The model under review builds one solid part; all positions refer to its coordinate system, in mm. Round coordinates to 2 decimals unless told otherwise and drop trailing zeros. Write each loop counter-clockwise with the first axis right and the second up, starting at its lowest first coordinate (ties: lowest second). Pieces come first, ordered by that corner, then holes. Notation, with made-up numbers: (-36.5, 46.25) -> (-15.5, 46.25) arc R16 ccw to (-15.5, 75.25) -> close; hole circle Ø1 at (-21.75, 8). An arc over 180 degrees is marked (long way). Use CSV: the item, a comma, the result in double quotes. Start each with the question number.
1) Take a section at B-B, the plane x = 504. Give the boundary of the cut face in (y, z).
2) For pin 1 Ø4 at (x, y) = (20, 60) entering from -Z; pin 2 Ø7 at (x, y) = (517, 269) entering from +Z; pin 3 Ø5 at (x, y) = (91, 15) entering from +Z; pin 4 Ø5.5 at (x, y) = (375, 15) entering from +Z, all flat-tipped, find the tip position at first contact; note any pin that passes through.
3) Wall thickness on probe 1 along X at (y, z) = (231.5, 0.6); probe 2 along Y at (x, z) = (20, 0.35); probe 3 along X at (y, z) = (224, 0.6): over which ranges is each line inside the solid? List them lowest first. Write a range as [from, to].
4) Take a section at A-A, the plane y = 205.5. Give the boundary of the cut face in (x, z), then the cut area to 3 significant figures.
from build123d import *

# Parameters (mm, degrees)
SKETCH_1_W                  = 750
SKETCH_1_H                  = 284
SKETCH_1_W_2                = 320
SKETCH_1_H_2                = 220
SKETCH_1_W_3                = 20
EXTRUDE_1_DEPTH             = 3
HOLE_WIZARD_M41_AT_2_COUNT  = 2
HOLE_WIZARD_M41_AT_2_PITCH  = 254
HOLE_WIZARD_M41_AT_3_COUNT  = 2
HOLE_WIZARD_M41_AT_3_PITCH  = 71
HOLE_WIZARD_M41_AT_4_COUNT  = 2
HOLE_WIZARD_M41_AT_4_PITCH  = 263.736611035
HOLE_WIZARD_M41_AT_5_COUNT  = 2
HOLE_WIZARD_M41_AT_5_PITCH  = 142
HOLE_WIZARD_M41_AT_6_COUNT  = 2
HOLE_WIZARD_M41_AT_6_PITCH  = 290.998281782
HOLE_WIZARD_M41_AT_7_COUNT  = 2
HOLE_WIZARD_M41_AT_7_PITCH  = 213
HOLE_WIZARD_M41_AT_8_COUNT  = 2
HOLE_WIZARD_M41_AT_8_PITCH  = 331.489064676
HOLE_WIZARD_M41_AT_9_COUNT  = 2
HOLE_WIZARD_M41_AT_9_PITCH  = 284
HOLE_WIZARD_M41_AT_10_COUNT = 2
HOLE_WIZARD_M41_AT_10_PITCH = 381.014435422
HOLE_WIZARD_M41_AT_11_COUNT = 2
HOLE_WIZARD_M41_AT_11_PITCH = 355
HOLE_WIZARD_M41_AT_12_COUNT = 2
HOLE_WIZARD_M41_AT_12_PITCH = 436.510022794
HOLE_WIZARD_M41_AT_13_COUNT = 2
HOLE_WIZARD_M41_AT_13_PITCH = 426
HOLE_WIZARD_M41_AT_14_COUNT = 2
HOLE_WIZARD_M41_AT_14_PITCH = 495.975805862
HOLE_WIZARD_M41_AT_15_COUNT = 2
HOLE_WIZARD_M41_AT_15_PITCH = 497
HOLE_WIZARD_M41_AT_16_COUNT = 2
HOLE_WIZARD_M41_AT_16_PITCH = 558.144246589
HOLE_WIZARD_M41_AT_17_COUNT = 2
HOLE_WIZARD_M41_AT_17_PITCH = 568
HOLE_WIZARD_M41_AT_18_COUNT = 2
HOLE_WIZARD_M41_AT_18_PITCH = 622.20575375
HOLE_WIZARD_M41_AT_19_COUNT = 2
HOLE_WIZARD_M41_AT_19_PITCH = 639
HOLE_WIZARD_M41_AT_20_COUNT = 2
HOLE_WIZARD_M41_AT_20_PITCH = 687.63144198
HOLE_WIZARD_M41_AT_21_COUNT = 2
HOLE_WIZARD_M41_AT_21_PITCH = 710
HOLE_WIZARD_M41_AT_22_COUNT = 2
HOLE_WIZARD_M41_AT_22_PITCH = 754.066310082
HOLE_WIZARD_M42_AT_2_COUNT  = 2
HOLE_WIZARD_M42_AT_2_PITCH  = 710
HOLE_WIZARD_M42_AT_3_COUNT  = 2
HOLE_WIZARD_M42_AT_3_PITCH  = 82
HOLE_WIZARD_M42_AT_4_COUNT  = 2
HOLE_WIZARD_M42_AT_4_PITCH  = 714.719525408
HOLE_WIZARD_M42_AT_5_COUNT  = 2
HOLE_WIZARD_M42_AT_5_PITCH  = 164
HOLE_WIZARD_M42_AT_6_COUNT  = 2
HOLE_WIZARD_M42_AT_6_PITCH  = 728.694723461


with BuildPart() as part:
    # Эскиз1 → Бобышка-Вытянуть1 (new body)
    with BuildSketch(Plane.XY):
        with Locations((375, 142)):
            Rectangle(SKETCH_1_W, SKETCH_1_H)
        with Locations((383, 142)):
            Rectangle(SKETCH_1_W_2, SKETCH_1_H_2, mode=Mode.SUBTRACT)
        with Locations((198, 142)):
            Rectangle(SKETCH_1_W_3, SKETCH_1_H_2, mode=Mode.SUBTRACT)
    extrude(amount=EXTRUDE_1_DEPTH)

    # Эскиз2 → Зенковка для винта с полупотайной головкой M41 (revolve, cut)
    with BuildSketch(Plane(origin=(20, 15, 3), x_dir=(0, -1, 0), z_dir=(1, 0, 0))):
        Polygon((0, 0), (0, 3), (2.15, 3), (2.15, 2.15), (4.3, 0), align=None)
    hole_wizard_m41 = revolve(axis=Axis((20, 15, 9.35), (0, 0, -1)), mode=Mode.SUBTRACT)

    # Зенковка для винта с полупотайной головкой M41 at 2: Зенковка для винта с полупотайной головкой M41 ×2
    with Locations(*[(0, i * HOLE_WIZARD_M41_AT_2_PITCH, 0) for i in range(1, HOLE_WIZARD_M41_AT_2_COUNT)]):
        add(hole_wizard_m41, mode=Mode.SUBTRACT)

    # Зенковка для винта с полупотайной головкой M41 at 3: Зенковка для винта с полупотайной головкой M41 ×2
    with Locations(*[(i * HOLE_WIZARD_M41_AT_3_PITCH, 0, 0) for i in range(1, HOLE_WIZARD_M41_AT_3_COUNT)]):
        add(hole_wizard_m41, mode=Mode.SUBTRACT)

    # Зенковка для винта с полупотайной головкой M41 at 4: Зенковка для винта с полупотайной головкой M41 ×2
    with Locations(*[Vector(0.2692079788296573, 0.9630820651089143, 0) * (i * HOLE_WIZARD_M41_AT_4_PITCH) for i in range(1, HOLE_WIZARD_M41_AT_4_COUNT)]):
        add(hole_wizard_m41, mode=Mode.SUBTRACT)

    # Зенковка для винта с полупотайной головкой M41 at 5: Зенковка для винта с полупотайной головкой M41 ×2
    with Locations(*[(i * HOLE_WIZARD_M41_AT_5_PITCH, 0, 0) for i in range(1, HOLE_WIZARD_M41_AT_5_COUNT)]):
        add(hole_wizard_m41, mode=Mode.SUBTRACT)

    # Зенковка для винта с полупотайной головкой M41 at 6: Зенковка для винта с полупотайной головкой M41 ×2
    with Locations(*[Vector(0.4879753898562281, 0.8728573874893093, 0) * (i * HOLE_WIZARD_M41_AT_6_PITCH) for i in range(1, HOLE_WIZARD_M41_AT_6_COUNT)]):
        add(hole_wizard_m41, mode=Mode.SUBTRACT)

    # Зенковка для винта с полупотайной головкой M41 at 7: Зенковка для винта с полупотайной головкой M41 ×2
    with Locations(*[(i * HOLE_WIZARD_M41_AT_7_PITCH, 0, 0) for i in range(1, HOLE_WIZARD_M41_AT_7_COUNT)]):
        add(hole_wizard_m41, mode=Mode.SUBTRACT)

    # Зенковка для винта с полупотайной головкой M41 at 8: Зенковка для винта с полупотайной головкой M41 ×2
    with Locations(*[Vector(0.6425551328758441, 0.7662394542275323, 0) * (i * HOLE_WIZARD_M41_AT_8_PITCH) for i in range(1, HOLE_WIZARD_M41_AT_8_COUNT)]):
        add(hole_wizard_m41, mode=Mode.SUBTRACT)

    # Зенковка для винта с полупотайной головкой M41 at 9: Зенковка для винта с полупотайной головкой M41 ×2
    with Locations(*[(i * HOLE_WIZARD_M41_AT_9_PITCH, 0, 0) for i in range(1, HOLE_WIZARD_M41_AT_9_COUNT)]):
        add(hole_wizard_m41, mode=Mode.SUBTRACT)

    # Зенковка для винта с полупотайной головкой M41 at 10: Зенковка для винта с полупотайной головкой M41 ×2
    with Locations(*[Vector(0.7453785830591875, 0.6666414087923718, 0) * (i * HOLE_WIZARD_M41_AT_10_PITCH) for i in range(1, HOLE_WIZARD_M41_AT_10_COUNT)]):
        add(hole_wizard_m41, mode=Mode.SUBTRACT)

    # Зенковка для винта с полупотайной головкой M41 at 11: Зенковка для винта с полупотайной головкой M41 ×2
    with Locations(*[(i * HOLE_WIZARD_M41_AT_11_PITCH, 0, 0) for i in range(1, HOLE_WIZARD_M41_AT_11_COUNT)]):
        add(hole_wizard_m41, mode=Mode.SUBTRACT)

    # Зенковка для винта с полупотайной головкой M41 at 12: Зенковка для винта с полупотайной головкой M41 ×2
    with Locations(*[Vector(0.8132688402602337, 0.5818881279608432, 0) * (i * HOLE_WIZARD_M41_AT_12_PITCH) for i in range(1, HOLE_WIZARD_M41_AT_12_COUNT)]):
        add(hole_wizard_m41, mode=Mode.SUBTRACT)

    # Зенковка для винта с полупотайной головкой M41 at 13: Зенковка для винта с полупотайной головкой M41 ×2
    with Locations(*[(i * HOLE_WIZARD_M41_AT_13_PITCH, 0, 0) for i in range(1, HOLE_WIZARD_M41_AT_13_COUNT)]):
        add(hole_wizard_m41, mode=Mode.SUBTRACT)

    # Зенковка для винта с полупотайной головкой M41 at 14: Зенковка для винта с полупотайной головкой M41 ×2
    with Locations(*[Vector(0.8589128642273502, 0.5121217547271055, 0) * (i * HOLE_WIZARD_M41_AT_14_PITCH) for i in range(1, HOLE_WIZARD_M41_AT_14_COUNT)]):
        add(hole_wizard_m41, mode=Mode.SUBTRACT)

    # Зенковка для винта с полупотайной головкой M41 at 15: Зенковка для винта с полупотайной головкой M41 ×2
    with Locations(*[(i * HOLE_WIZARD_M41_AT_15_PITCH, 0, 0) for i in range(1, HOLE_WIZARD_M41_AT_15_COUNT)]):
        add(hole_wizard_m41, mode=Mode.SUBTRACT)

    # Зенковка для винта с полупотайной головкой M41 at 16: Зенковка для винта с полупотайной головкой M41 ×2
    with Locations(*[Vector(0.8904508163214954, 0.4550794916411667, 0) * (i * HOLE_WIZARD_M41_AT_16_PITCH) for i in range(1, HOLE_WIZARD_M41_AT_16_COUNT)]):
        add(hole_wizard_m41, mode=Mode.SUBTRACT)

    # Зенковка для винта с полупотайной головкой M41 at 17: Зенковка для винта с полупотайной головкой M41 ×2
    with Locations(*[(i * HOLE_WIZARD_M41_AT_17_PITCH, 0, 0) for i in range(1, HOLE_WIZARD_M41_AT_17_COUNT)]):
        add(hole_wizard_m41, mode=Mode.SUBTRACT)

    # Зенковка для винта с полупотайной головкой M41 at 18: Зенковка для винта с полупотайной головкой M41 ×2
    with Locations(*[Vector(0.912881304257323, 0.4082250902840845, 0) * (i * HOLE_WIZARD_M41_AT_18_PITCH) for i in range(1, HOLE_WIZARD_M41_AT_18_COUNT)]):
        add(hole_wizard_m41, mode=Mode.SUBTRACT)

    # Зенковка для винта с полупотайной головкой M41 at 19: Зенковка для винта с полупотайной головкой M41 ×2
    with Locations(*[(i * HOLE_WIZARD_M41_AT_19_PITCH, 0, 0) for i in range(1, HOLE_WIZARD_M41_AT_19_COUNT)]):
        add(hole_wizard_m41, mode=Mode.SUBTRACT)

    # Зенковка для винта с полупотайной головкой M41 at 20: Зенковка для винта с полупотайной головкой M41 ×2
    with Locations(*[Vector(0.9292768785553057, 0.36938392355719507, 0) * (i * HOLE_WIZARD_M41_AT_20_PITCH) for i in range(1, HOLE_WIZARD_M41_AT_20_COUNT)]):
        add(hole_wizard_m41, mode=Mode.SUBTRACT)

    # Зенковка для винта с полупотайной головкой M41 at 21: Зенковка для винта с полупотайной головкой M41 ×2
    with Locations(*[(i * HOLE_WIZARD_M41_AT_21_PITCH, 0, 0) for i in range(1, HOLE_WIZARD_M41_AT_21_COUNT)]):
        add(hole_wizard_m41, mode=Mode.SUBTRACT)

    # Зенковка для винта с полупотайной головкой M41 at 22: Зенковка для винта с полупотайной головкой M41 ×2
    with Locations(*[Vector(0.9415617572454846, 0.3368404032962719, 0) * (i * HOLE_WIZARD_M41_AT_22_PITCH) for i in range(1, HOLE_WIZARD_M41_AT_22_COUNT)]):
        add(hole_wizard_m41, mode=Mode.SUBTRACT)

    # Эскиз4 → Зенковка для винта с полупотайной головкой M42 (revolve, cut)
    with BuildSketch(Plane(origin=(20, 224, 3), x_dir=(0, -1, 0), z_dir=(1, 0, 0))):
        Polygon((0, 0), (0, 3), (2.25, 3), (2.25, 2.05), (4.3, 0), align=None)
    hole_wizard_m42 = revolve(axis=Axis((20, 224, 9.35), (0, 0, -1)), mode=Mode.SUBTRACT)

    # Зенковка для винта с полупотайной головкой M42 at 2: Зенковка для винта с полупотайной головкой M42 ×2
    with Locations(*[(i * HOLE_WIZARD_M42_AT_2_PITCH, 0, 0) for i in range(1, HOLE_WIZARD_M42_AT_2_COUNT)]):
        add(hole_wizard_m42, mode=Mode.SUBTRACT)

    # Зенковка для винта с полупотайной головкой M42 at 3: Зенковка для винта с полупотайной головкой M42 ×2
    with Locations(*[(0, -i * HOLE_WIZARD_M42_AT_3_PITCH, 0) for i in range(1, HOLE_WIZARD_M42_AT_3_COUNT)]):
        add(hole_wizard_m42, mode=Mode.SUBTRACT)

    # Зенковка для винта с полупотайной головкой M42 at 4: Зенковка для винта с полупотайной головкой M42 ×2
    with Locations(*[Vector(0.9933966748624963, -0.11473032019538675, 0) * (i * HOLE_WIZARD_M42_AT_4_PITCH) for i in range(1, HOLE_WIZARD_M42_AT_4_COUNT)]):
        add(hole_wizard_m42, mode=Mode.SUBTRACT)

    # Зенковка для винта с полупотайной головкой M42 at 5: Зенковка для винта с полупотайной головкой M42 ×2
    with Locations(*[(0, -i * HOLE_WIZARD_M42_AT_5_PITCH, 0) for i in range(1, HOLE_WIZARD_M42_AT_5_COUNT)]):
        add(hole_wizard_m42, mode=Mode.SUBTRACT)

    # Зенковка для винта с полупотайной головкой M42 at 6: Зенковка для винта с полупотайной головкой M42 ×2
    with Locations(*[Vector(0.9743449172072053, -0.22505995270701593, 0) * (i * HOLE_WIZARD_M42_AT_6_PITCH) for i in range(1, HOLE_WIZARD_M42_AT_6_COUNT)]):
        add(hole_wizard_m42, mode=Mode.SUBTRACT)


solid = part.part
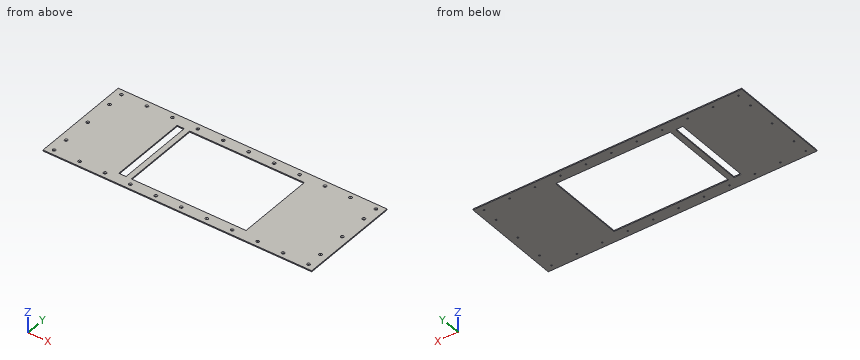
Values found:
1,outline,"(0, 0) -> (32, 0) -> (32, 3) -> (0, 3) -> close; (252, 0) -> (284, 0) -> (284, 3) -> (252, 3) -> close"
2,pin 1,"through"
2,pin 2,"z = 2.2"
2,pin 3,"z = 1.2"
2,pin 4,"z = 1.45"
3,probe 1,"[0, 188], [208, 223], [543, 750]"
3,probe 2,"[0, 12.85], [17.15, 57.75], [62.25, 139.75], [144.25, 221.75], [226.25, 266.85], [271.15, 284]"
3,probe 3,"[0, 17.75], [22.25, 188], [208, 223], [543, 727.75], [732.25, 750]"
4,outline,"(0, 0) -> (188, 0) -> (188, 3) -> (0, 3) -> close; (208, 0) -> (223, 0) -> (223, 3) -> (208, 3) -> close; (543, 0) -> (750, 0) -> (750, 3) -> (543, 3) -> close"
4,area,"1,230 mm²"
